Can you work these out from the model? Positions are in its coordinate system, mm. A direction names the side the tool comes from. Give positions to 0.01 mm unless a question says otherwise; leave off trailing zeros. Write each loop counter-clockwise with the first axis right and the second up, starting at its lowest first coordinate (ties: lowest second). Pieces come first, ordered by that corner, then holes.
from build123d import *

# Parameters (mm, degrees)
SKETCH_1_R      = 1.6
EXTRUDE_1_DEPTH = 1.5
FILLET_5_R      = 3
FILLET_6_R      = 5
FILLET_8_R      = 10


with BuildPart() as part:
    # ｽｹｯﾁ1 → ﾎﾞｽ - 押し出し1 (new body)
    with BuildSketch(Plane.XY):
        Polygon((16.25, -10.3), (16.25, 10.3), (-11.25, 10.3), (-18.25, 25), (-28.25, 25), (-28.25, 4.9), (-16.25, 4.9), (-16.25, -10.3), align=None)
        with Locations((-11.25, -5.3)):
            Circle(SKETCH_1_R, mode=Mode.SUBTRACT)
        with Locations((11.25, -5.3)):
            Circle(SKETCH_1_R, mode=Mode.SUBTRACT)
        with Locations((-11.25, 5.3)):
            Circle(SKETCH_1_R, mode=Mode.SUBTRACT)
        with Locations((11.25, 5.3)):
            Circle(SKETCH_1_R, mode=Mode.SUBTRACT)
        with Locations((-23.25, 20)):
            Circle(SKETCH_1_R, mode=Mode.SUBTRACT)
        with Locations((-23.25, 10)):
            Circle(SKETCH_1_R, mode=Mode.SUBTRACT)
    extrude(amount=EXTRUDE_1_DEPTH)

    # ﾌｨﾚｯﾄ5
    fillet_5_edges = [part.edges().sort_by_distance(p)[0] for p in [
        (-28.25, 4.9, 0.75),
        (-28.25, 25, 0.75),
        (-18.25, 25, 0.75),
        (16.25, 10.3, 0.75),
        (16.25, -10.3, 0.75),
        (-16.25, -10.3, 0.75),
    ]]
    fillet(fillet_5_edges, radius=FILLET_5_R)

    # ﾌｨﾚｯﾄ6
    fillet_6_edges = [part.edges().sort_by_distance(p)[0] for p in [
        (-16.25, 4.9, 0.75),
    ]]
    fillet(fillet_6_edges, radius=FILLET_6_R)

    # ﾌｨﾚｯﾄ8
    fillet_8_edges = [part.edges().sort_by_distance(p)[0] for p in [
        (-11.25, 10.3, 0.75),
    ]]
    fillet(fillet_8_edges, radius=FILLET_8_R)


solid = part.part
(1) For faces 4 (the face through (4, 10.3, 1)), 5 (the face through (-23, 4.9, 1)), 6 (the face through (15.39, -9.4, 0.76)), which set-ups out of +Z, -Z, +X, -X, +Y, -Y let a thin tool reach every point of the face, with its end or its side?
Returned:
face 4: +Z, -Z, +X, +Y
face 5: +Z, -Z, -X, -Y
face 6: +Z, -Z, +X, -Y
(2) Will this pin go through, and if not, where does the flat tip stop? P1, Ø2.5, axis at x = -11.25, y = -5.3, coming from the +Z side.
Returned:
P1: passes through
(3) Imagine slicing it at D-D, the plane y = 20. Write out the boundary of the cut face in (x, z), plus the area to 3 significant figures.
Returned:
outline: (-28.25, 0) - (-24.85, 0) - (-24.85, 1.5) - (-28.25, 1.5) - close; (-21.65, 0) - (-15.87, 0) - (-15.87, 1.5) - (-21.65, 1.5) - close
area: 13.8 mm2
(4) If I drill on L1, parallel to Y at x = 11.25, z = 1.05; L2, parallel to Y at x = -24, z = 0.55; L3, parallel to Y at x = 8.5, z = 1.3, over which ranges is the centre line in solid material (lowest first)?
Returned:
L1: y = -10.3 to -6.9, -3.7 to 3.7, 6.9 to 10.3
L2: y = 4.9 to 8.59, 11.41 to 18.59, 21.41 to 25
L3: y = -10.3 to 10.3
(5) If we mould it in two halves opening along Y, with no side actions, what happens to faces 1 (the face through (-18.52, 24.52, 0.76)), 2 (the face through (-17.68, 3.4, 0.76)), 3 (the face through (-12.85, -5.23, 0.74))? For each: +Y half, -Y half, draft (parallel to the pull), parting line (faces both ways), or undercut.
Returned:
face 1: +Y half
face 2: -Y half
face 3: undercut
(6) Imagine slicing it at C-C, the plane y = -5.3. Write out the boundary of the cut face in (x, z), plus the area to 4 significant figures.
Returned:
outline: (-16.25, 0) - (-12.85, 0) - (-12.85, 1.5) - (-16.25, 1.5) - close; (-9.65, 0) - (9.65, 0) - (9.65, 1.5) - (-9.65, 1.5) - close; (12.85, 0) - (16.25, 0) - (16.25, 1.5) - (12.85, 1.5) - close
area: 39.15 mm2
(7) Imagine slicing it at B-B, the plane z = 1. Write out the boundary of the cut face in (x, y).
Returned:
outline: (-28.25, 7.9) arc R3 ccw to (-25.25, 4.9) - (-21.25, 4.9) arc R5 cw to (-16.25, -0.1) - (-16.25, -7.3) arc R3 ccw to (-13.25, -10.3) - (13.25, -10.3) arc R3 ccw to (16.25, -7.3) - (16.25, 7.3) arc R3 ccw to (13.25, 10.3) - (-4.94, 10.3) arc R10 cw to (-13.96, 16) - (-17.44, 23.29) arc R3 ccw to (-20.14, 25) - (-25.25, 25) arc R3 ccw to (-28.25, 22) - close; hole circle Ø3.2 at (-23.25, 10); hole circle Ø3.2 at (-23.25, 20); hole circle Ø3.2 at (-11.25, -5.3); hole circle Ø3.2 at (-11.25, 5.3); hole circle Ø3.2 at (11.25, -5.3); hole circle Ø3.2 at (11.25, 5.3)
(8) Imagine slicing it at A-A, the plane x = -23.25. Write out the boundary of the cut face in (y, z), plus the area to 4 significant figures.
Returned:
outline: (4.9, 0) - (8.4, 0) - (8.4, 1.5) - (4.9, 1.5) - close; (11.6, 0) - (18.4, 0) - (18.4, 1.5) - (11.6, 1.5) - close; (21.6, 0) - (25, 0) - (25, 1.5) - (21.6, 1.5) - close
area: 20.55 mm2
